Build history of the part. All positions in model axes, mm. A direction names the side the tool comes from. Give positions to 0.01 mm unless a question says otherwise; leave off trailing zeros. Write each loop counter-clockwise with the first axis right and the second up, starting at its lowest first coordinate (ties: lowest second). Pieces come first, ordered by that corner, then holes. Notation, with made-up numbers: M 9,3 L 65,3 A11 cw 65,9 Z; hole C 88.5,15 d2. An arc over 180 degrees is marked long. Return JSON: item names as keys, results as strings. Group by question number.
Q1. Tool access for faces 4 (the flat face through (1.3, 12, 1.3)), 5 (the cylindrical face through (-3, 13, 0)): list every direction of +Z, -Z, +X, -X, +Y, -Y with a clear straight run to the whole face (end or side of a thin tool).
Q2. Pull direction X, two halves, no side cores. Call faces 1 (the flat face through (0, 0, 0)), 2 (the cylindrical face through (1.5, 5.92, -0.07)), 3 (the flat face through (0, 14.5, 0)): +X half, -X half, draft (parallel to the pull), parting line (faces both ways), or undercut.
Q3. Band-saw the part on A-A, the plane x = 0. Give the cut face in (y, z), then the cut area to 3 significant figures.
Q4. Band-saw the part on D-D, the plane z = 2.15. Give the cut face in (x, y).
Q5. Wall check: probe 1 along Y at (x, z) = (-1.7, -0.15); probe 2 along Y at (x, z) = (-1.9, 1.4); probe 3 along X at (y, z) = (3, -0.1). Give the ranges that are in metal, low to high.
Q6. Band-saw the part on C-C, the plane y = 6. Give the cut face in (x, z), then the cut area to 3 significant figures.
Q7. Band-saw the part on B-B, the plane z = 0. Give the cut face in (x, y).
Q8. Flat gauge pins, fed straight in: pin 1 Ø0.6 at (x, y) = (-1.5, 14.5) entering from +Z; pin 2 Ø2 at (y, z) = (6.5, 1.5) entering from +X; pin 3 Ø0.6 at (y, z) = (15, 1) entering from -X. Where does each tip first touch, or does it go through?
Autodesk Inventor part; units mm, degrees
ref_plane "YZ Plane" through (0, 0, 0) normal (1, 0, 0) x (0, 1, 0)
ref_plane "XZ Plane" through (0, 0, 0) normal (0, 1, 0) x (-1, 0, 0)
ref_plane "XY Plane" through (0, 0, 0) normal (0, 0, 1) x (1, 0, 0)
sketch "Sketch1" plane through (0, 0, 0) normal (0, 1, 0) x (-1, 0, 0)
  circle A0 centre (0, 0) radius 1.5
  dimension "d0" = 3
extrude "Extrusion1" add sketch "Sketch1" along normal blind 12
sketch "Sketch2" plane through (0, 12, 0) normal (0, 1, 0) x (1, 0, 0)
  circle A0 centre (0, 0) radius 3
  dimension "d3" = 6
extrude "Extrusion2" add sketch "Sketch2" along normal blind 3
sketch "Sketch3" plane through (0, 15, 0) normal (0, 1, 0) x (1, 0, 0)
  line L0 (-2, -0.3) -> (-0.3, -0.3)
  line L1 (-0.3, -0.3) -> (-0.3, -2)
  line L2 (-0.3, -2) -> (0.3, -2)
  line L3 (0.3, -2) -> (0.3, -0.3)
  line L4 (0.3, -0.3) -> (2, -0.3)
  line L5 (2, -0.3) -> (2, 0.3)
  line L6 (2, 0.3) -> (0.3, 0.3)
  line L7 (0.3, 0.3) -> (0.3, 2)
  line L8 (0.3, 2) -> (-0.3, 2)
  line L9 (-0.3, 2) -> (-0.3, 0.3)
  line L10 (-2, 0.3) -> (-2, -0.3)
  line L11 (-2, 0.3) -> (-0.3, 0.3)
  circle A0 centre (0, 0) radius 3
  point P0 (0, 0)
  dimension "d19" = 0.3
  dimension "d20" = 0.3
  dimension "d22" = 2
  dimension "d23" = 0
  dimension "d26" = 0.3
  dimension "d27" = 0.3
extrude "Extrusion3" cut sketch "Sketch3" against normal blind 0.5 contours L10 L11 L9 L8 L7 L6 L5 L4 L3 L2 L1 L0
thread "Thread1"
properties part number "BoltM3-PI" material "PC/ABS Plastic"
From the geometry:
{
 "1": {"face 4": "-Y", "face 5": "+Y, -Y"},
 "2": {"face 1": "draft", "face 2": "parting line", "face 3": "undercut"},
 "3": {"outline": "M 0,-1.5 L 12,-1.5 L 12,-3 L 15,-3 L 15,-2 L 14.5,-2 L 14.5,2 L 15,2 L 15,3 L 12,3 L 12,1.5 L 0,1.5 Z", "area": "52.0 mm^2"},
 "4": {"outline": "M -2.09,12 L 2.09,12 L 2.09,15 L -2.09,15 Z"},
 "5": {"probe 1": "y = 12 to 14.5", "probe 2": "y = 12 to 15", "probe 3": "x = -1.5 to 1.5"},
 "6": {"outline": "C 0,0 d3", "area": "7.07 mm^2"},
 "7": {"outline": "M -3,12 L -1.5,12 L -1.5,0 L 1.5,0 L 1.5,12 L 3,12 L 3,15 L 2,15 L 2,14.5 L -2,14.5 L -2,15 L -3,15 Z"},
 "8": {"pin 1": "stops at z = 2.75", "pin 2": "stops at x = 1.41", "pin 3": "stops at x = -2.92"}
}
